For this review, take the finished solid that the model builds, in its own axes (mm). Face numbers are marked on the shaded views. A direction names the side the tool comes from. Round coordinates to 2 decimals unless told otherwise and drop trailing zeros. Order: outer loops, then holes, each group sorted by start corner. A loop starts at its lowest first (then second) coordinate and runs counter-clockwise, first axis right, second up. Notation, with made-up numbers: (68, -4) -> (124, -4) arc R30 cw to (124, 31) -> close; hole circle Ø2 at (-40, 54). An arc over 180 degrees is marked (long way). Use a Markdown table: item, result. Add a question column.
1) Consider section C-C (x = -12). State the section outline as (y, z) points, plus the area to 3 significant figures.
2) Wall thickness on line 1 along Z through (x, y) = (9, 6.5); line 2 along X through (y, z) = (6.3, 0) (3 decimals); line 3 along Z through (x, y) = (11, 6): over which ranges is each line inside the solid? List them lowest first. Write a range as [from, to].
3) Clearance check with flat-ended pins moving along their axes: P1, Ø6, axis at x = -7.5, z = 3.5, coming from the +Y side; P2, Ø4, axis at x = 7.5, y = 6, coming from the +Z side; P3, Ø4, axis at x = 12.5, z = 4, coming from the +Y side. State where each tip first meets the part, or that it passes through.
4) Consider section A-A (y = 6.5). State the section outline as (x, z) points (3 decimals), plus the area to 3 significant figures.
5) Draft analysis for pull direction X (two halves, no side actions). For the marked faces 1, 2 and 3, state which applies: pulls with the +X half, pulls with the -X half, needs draft (parallel to the pull), parting line crosses it, or undercut.
6) Consider section D-D (x = 1.5). State the section outline as (y, z) points, plus the area to 3 significant figures.
7) Machinability: for the marked faces 4, 5, 6 and 7, which of the approach directions +Z, -Z, +X, -X, +Y, -Y give a long, thin tool a straight path to every point of the face, cutting with its end or side? Answer none if there is none.
```python
from build123d import *

# Parameters (mm, degrees)
SKETCH1_W                  = 33.02
SKETCH1_H                  = 10.414
BOSS_EXTRUDE1_DEPTH        = 1.6
SKETCH2_R                  = 1.6
CUT_EXTRUDE1_DEPTH         = 18.385423463
SKETCH3_W                  = 22
SKETCH3_H                  = 8
BOSS_EXTRUDE2_DEPTH        = 7.52
SKETCH5_R                  = 3.335
CUT_EXTRUDE2_DEPTH         = 5
SKETCH6_R                  = 2.334999968
BOSS_EXTRUDE3_DEPTH        = 3
DOME1_FACE_RADIUS          = 2.334999968
DOME1_HEIGHT               = 2.54
MIRROR1_COPY_1_FACE_RADIUS = 2.334999968
MIRROR1_COPY_1_HEIGHT      = 2.54
SKETCH7_W                  = 4.77
SKETCH7_H                  = 6.139999912
CUT_EXTRUDE3_DEPTH         = 1


with BuildPart() as part:
    # Sketch1 → Boss-Extrude1 (new body)
    with BuildSketch(Plane(origin=(0, 0, 0), x_dir=(1, 0, 0), z_dir=(0, 1, 0))):
        Rectangle(SKETCH1_W, SKETCH1_H)
    extrude(amount=BOSS_EXTRUDE1_DEPTH)

    # Sketch2 → Cut-Extrude1 (cut, through all)
    with BuildSketch(Plane(origin=(0, 1.6, 0), x_dir=(1, 0, 0), z_dir=(0, 1, 0))):
        with Locations(Location((-12.7, 0, 0), (0, 0, 270))):
            Circle(SKETCH2_R)
    extrude(amount=-CUT_EXTRUDE1_DEPTH, mode=Mode.SUBTRACT)

    # Sketch3 → Boss-Extrude2 (add)
    with BuildSketch(Plane(origin=(0, 1.6, 0), x_dir=(1, 0, 0), z_dir=(0, 1, 0))):
        with Locations((2.16, 0)):
            Rectangle(SKETCH3_W, SKETCH3_H)
    extrude(amount=BOSS_EXTRUDE2_DEPTH)

    # Sketch5 → Cut-Extrude2 (cut)
    with BuildSketch(Plane(origin=(0, 9.12, 0), x_dir=(1, 0, 0), z_dir=(0, 1, 0))):
        with Locations(Location((-4.84, 0, 0), (0, 0, 270))):
            Circle(SKETCH5_R)
        with Locations(Location((9.16, 0, 0), (0, 0, 90))):
            Circle(SKETCH5_R)
    extrude(amount=-CUT_EXTRUDE2_DEPTH, mode=Mode.SUBTRACT)

    # Sketch6 → Boss-Extrude3 (add)
    with BuildSketch(Plane(origin=(0, 4.12, 0), x_dir=(1, 0, 0), z_dir=(0, 1, 0))):
        with Locations(Location((-4.84, 0, 0), (0, 0, 270))):
            Circle(SKETCH6_R)
    boss_extrude3 = extrude(amount=BOSS_EXTRUDE3_DEPTH)

    # Dome1: a dome of height H over a round flat face of radius A is a cap of a sphere of radius (A * A + H * H) / (2 * H)
    dome1_r = (DOME1_FACE_RADIUS * DOME1_FACE_RADIUS + DOME1_HEIGHT * DOME1_HEIGHT) / (2 * DOME1_HEIGHT)
    dome1_base = Plane((-4.84, 7.12, 0), z_dir=(0, 1, 0))
    with Locations(dome1_base.offset(DOME1_HEIGHT - dome1_r)):
        dome1_ball = Sphere(dome1_r, mode=Mode.PRIVATE)
    add(split(dome1_ball, bisect_by=dome1_base, keep=Keep.TOP, mode=Mode.PRIVATE))

    # Mirror1: Boss-Extrude3 across plane
    add(boss_extrude3.mirror(Plane(origin=(2.16, 0, 0), x_dir=(0, 0, 1), z_dir=(1, 0, 0))))

    # Mirror1 copy 1: a dome of height H over a round flat face of radius A is a cap of a sphere of radius (A * A + H * H) / (2 * H)
    mirror1_copy_1_r = (MIRROR1_COPY_1_FACE_RADIUS * MIRROR1_COPY_1_FACE_RADIUS + MIRROR1_COPY_1_HEIGHT * MIRROR1_COPY_1_HEIGHT) / (2 * MIRROR1_COPY_1_HEIGHT)
    mirror1_copy_1_base = Plane((9.16, 7.12, 0), z_dir=(0, 1, 0))
    with Locations(mirror1_copy_1_base.offset(MIRROR1_COPY_1_HEIGHT - mirror1_copy_1_r)):
        mirror1_copy_1_ball = Sphere(mirror1_copy_1_r, mode=Mode.PRIVATE)
    add(split(mirror1_copy_1_ball, bisect_by=mirror1_copy_1_base, keep=Keep.TOP, mode=Mode.PRIVATE))

    # Sketch7 → Cut-Extrude3 (cut)
    with BuildSketch(Plane(origin=(0, 9.12, 0), x_dir=(1, 0, 0), z_dir=(0, 1, 0))):
        with Locations((1.942220891, 0)):
            Rectangle(SKETCH7_W, SKETCH7_H)
    extrude(amount=-CUT_EXTRUDE3_DEPTH, mode=Mode.SUBTRACT)


solid = part.part
```
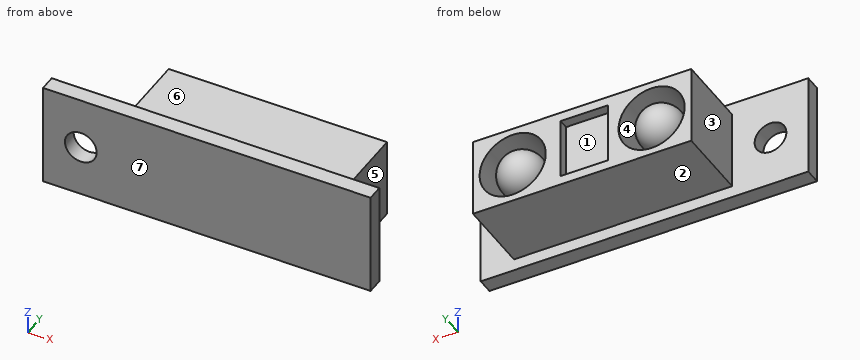
Results list:
| question | item | result |
|---|---|---|
| 1 | outline | (0, -5.21) -> (1.6, -5.21) -> (1.6, -1.44) -> (0, -1.44) -> close; (0, 1.44) -> (1.6, 1.44) -> (1.6, 5.21) -> (0, 5.21) -> close |
| 1 | area | 12.1 mm2 |
| 2 | line 1 | [-4, -3.33], [-2.33, 2.33], [3.33, 4] |
| 2 | line 2 | [-8.84, -8.175], [-7.175, -2.505], [-1.505, 5.825], [6.825, 11.495], [12.495, 13.16] |
| 2 | line 3 | [-4, -2.78], [-1.44, 1.44], [2.78, 4] |
| 3 | P1 | y = 9.2 |
| 3 | P2 | z = 4 |
| 3 | P3 | y = 9.12 |
| 4 | outline | (-8.84, -4) -> (13.16, -4) -> (13.16, 4) -> (-8.84, 4) -> close; circle Ø4.67 at (-4.84, 0); circle Ø4.67 at (9.16, 0); hole circle Ø6.67 at (-4.84, 0); hole circle Ø6.67 at (9.16, 0) |
| 4 | area | 140 mm2 |
| 5 | face 1 | undercut |
| 5 | face 2 | needs draft |
| 5 | face 3 | pulls with the -X half |
| 6 | outline | (0, -5.21) -> (1.6, -5.21) -> (1.6, -4) -> (9.12, -4) -> (9.12, -3.07) -> (8.12, -3.07) -> (8.12, 3.07) -> (9.12, 3.07) -> (9.12, 4) -> (1.6, 4) -> (1.6, 5.21) -> (0, 5.21) -> close |
| 6 | area | 70.7 mm2 |
| 7 | face 4 | +Y |
| 7 | face 5 | +Z, -Z, +X, +Y |
| 7 | face 6 | +Z, +X, -X, +Y |
| 7 | face 7 | +Z, -Z, +X, -X, -Y |
